Read the model definition and answer for the solid it produces. Units are mm, in the model's axes. Face numbers are marked on the shaded views. A direction names the side the tool comes from. Give positions to 0.01 mm unless a question says otherwise; leave off trailing zeros. Order: outer loops, then holes, each group sorted by start corner. A loop starts at its lowest first (then second) coordinate and runs counter-clockwise, first axis right, second up. Notation, with made-up numbers: (13.5, 77) -> (53.5, 77) arc R20 ccw to (53.5, 101) -> close; hole circle Ø6 at (62.5, -33.75). An arc over 180 degrees is marked (long way). One line per item, written item: value. Start each with the question number.
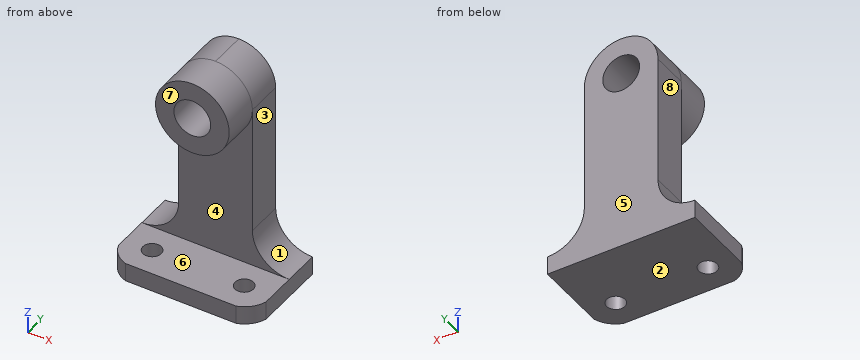
from build123d import *
from build123d import SkipClean  # not in build123d's __all__

# Parameters (mm, degrees)
F1_DEPTH  = 12.7
F2_W      = 50.8
F2_H      = 6.35
F3_DEPTH  = 19.05
F5_DEPTH  = 12.7
F7_R      = 12.7
F8_DEPTH  = 25.4
F9_R      = 6.35
F10_DEPTH = 25.4
F11_R     = 3.175
F12_DEPTH = 6.35


with BuildPart() as f1:
    # F0 (on Front) → F1 (new body)
    with BuildSketch(Plane.XZ):
        Polygon((0, 19.05), (0, 0), (50.8, 0), (50.8, 19.05), (38.1, 19.05), (38.1, 76.2), (12.7, 76.2), (12.7, 19.05), align=None)
    extrude(amount=F1_DEPTH)

    # F2 (on face) → F3 (join)
    with BuildSketch(Plane.XZ.offset(12.7)):
        with Locations((25.4, 3.175)):
            Rectangle(F2_W, F2_H)
    extrude(amount=F3_DEPTH)

    # F4 (on face) → F5 (cut)
    with BuildSketch(Plane.XZ.offset(12.7)):
        with BuildLine():
            Line((0, 19.05), (0, 6.35))
            ThreePointArc((0, 6.35), (8.9802561211, 10.0697438789), (12.7, 19.05))
            Line((12.7, 19.05), (0, 19.05))
        make_face()
        with BuildLine():
            Line((50.8, 19.05), (38.1, 19.05))
            ThreePointArc((38.1, 19.05), (41.8197438789, 10.0697438789), (50.8, 6.35))
            Line((50.8, 6.35), (50.8, 19.05))
        make_face()
    extrude(amount=-F5_DEPTH, mode=Mode.SUBTRACT)

    # F7 (on Front) → F8 (join)
    with BuildSketch(Plane.XZ):
        with Locations((25.4, 63.5)):
            Circle(F7_R)
    extrude(amount=F8_DEPTH)

    # F9 (on face) + F8_face1 (on face) → F10 (cut)
    with BuildSketch(Plane.XZ.offset(25.4)):
        with Locations((25.4, 63.5)):
            Circle(F9_R)
    with BuildSketch(Plane(origin=(35.2632271754, -12.7, 73.3632271754), x_dir=(1, 0, 0), z_dir=(0, -1, 0))):
        with BuildLine():
            Line((2.8367728246, -9.8632271754), (2.8367728246, 2.8367728246))
            Line((2.8367728246, 2.8367728246), (-9.8632271754, 2.8367728246))
            ThreePointArc((-9.8632271754, 2.8367728246), (-0.8829710543, -0.8829710543), (2.8367728246, -9.8632271754))
        make_face()
        with BuildLine():
            ThreePointArc((-22.5632271754, -9.8632271754), (-18.8434832965, -0.8829710543), (-9.8632271754, 2.8367728246))
            Line((-9.8632271754, 2.8367728246), (-22.5632271754, 2.8367728246))
            Line((-22.5632271754, 2.8367728246), (-22.5632271754, -9.8632271754))
        make_face()
    with SkipClean():  # cleaning this boolean's faces spoils the solid; the shape is the same uncleaned
        extrude(amount=-F10_DEPTH, mode=Mode.SUBTRACT)

    # F6 (on face) + F11 (on face) → F12 (cut)
    with BuildSketch(Plane.XY.offset(6.35)):
        with BuildLine():
            Line((0, -31.75), (6.35, -31.75))
            ThreePointArc((6.35, -31.75), (2.3796890107, -29.3703109893), (0, -25.4))
            Line((0, -25.4), (0, -31.75))
        make_face()
        with BuildLine():
            ThreePointArc((50.8, -25.4), (48.4203109893, -29.3703109893), (44.45, -31.75))
            Line((44.45, -31.75), (50.8, -31.75))
            Line((50.8, -31.75), (50.8, -25.4))
        make_face()
    with BuildSketch(Plane.XY.offset(6.35)):
        with Locations((9.525, -22.225)):
            Circle(F11_R)
        with Locations((41.275, -22.225)):
            Circle(F11_R)
    with SkipClean():  # cleaning this boolean's faces spoils the solid; the shape is the same uncleaned
        extrude(amount=-F12_DEPTH, mode=Mode.SUBTRACT)


solid = f1.part
Item 1: For a pull along Z with two mould halves and no side action, classify the marked faces 1, 2, 3 and 4 as +Z half, -Z half, draft (parallel to the pull), parting line (faces both ways), or undercut.
Item 2: Find section C-C on x = 45.5. Write down the section's boundary in (y, z).
Item 3: A tool of negligible diameter and unlimited length cuts with its end or side. For the marked faces 5, 6, 7 and 8, from which of +Z, -Z, +X, -X, +Y, -Y can it reach the whole face along a straight path? Write none if from no direction.
Item 4: Find the intervals of material crossed by line 1 (Z direction, x = 23, y = -20.5); line 2 (Z direction, x = 9, y = -14); line 3 (Z direction, x = 17, y = -19), in increasing order. Write a range as from..to.
Item 5: Find section A-A on y = -17. Write down the section's boundary in (x, z), then the cut area to 3 significant figures.
Item 6: Find section D-D on z = 9.5. Write down the section's boundary in (x, y), then the cut area to 3 significant figures.
Item 7: Find section B-B on x = 28.5. Write down the section's boundary in (y, z).
Item 8: Flat-ended cylindrical pins translate along their axes: pin 1 (8 mm diameter, centred on x = 13.5, z = 57.5, fed in from -Y); pin 2 (4 mm diameter, centred on y = -4, z = 52.5, fed in from +X); pin 3 (12 mm diameter, centred on y = -7.5, z = 44, fed in from -X). Find the tip coordinate at first contact, or state that the pin passes through.
Checks:
1. face 1: +Z half
1. face 2: -Z half
1. face 3: draft
1. face 4: undercut
2. outline: (-31.36, 0) -> (0, 0) -> (0, 7.51) -> (-12.7, 7.51) -> (-12.7, 6.35) -> (-31.36, 6.35) -> close
3. face 5: +Z, -Z, +X, -X, +Y
3. face 6: +X, -X, -Y
3. face 7: +Z, +X, -X, -Y
3. face 8: +Z, -X, +Y, -Y
4. line 1: 0..6.35, 51.03..57.62, 69.38..75.97
4. line 2: 0..6.35
4. line 3: 0..6.35, 53.97..73.03
5. outline: (0, 0) -> (50.8, 0) -> (50.8, 6.35) -> (0, 6.35) -> close; circle Ø25.4 at (25.4, 63.5); hole circle Ø12.7 at (25.4, 63.5)
5. area: 703 mm2
6. outline: (8.37, -12.7) -> (42.43, -12.7) -> (42.43, 0) -> (8.37, 0) -> close
6. area: 433 mm2
7. outline: (-31.75, 0) -> (0, 0) -> (0, 57.96) -> (-25.4, 57.96) -> (-25.4, 51.18) -> (-12.7, 51.18) -> (-12.7, 6.35) -> (-31.75, 6.35) -> close; (-25.4, 69.04) -> (0, 69.04) -> (0, 75.82) -> (-25.4, 75.82) -> close
8. pin 1: y = -25.4
8. pin 2: x = 38.1
8. pin 3: x = 12.7
